```python
from build123d import *
from build123d.topology import SkipClean

# Parameters (mm, degrees)
EXTRUDE1_DEPTH = 4
EXTRUDE2_DEPTH = 3
SKETCH4_R      = 1.5
EXTRUDE3_DEPTH = 4
FILLET3_R      = 3
EXTRUDE4_DEPTH = 4
EXTRUDE6_DEPTH = 3


with BuildPart() as part:
    # Sketch1 → Extrude1 (new body)
    with BuildSketch(Plane.XY):
        Polygon((0, 20.5), (0, 0), (-15, 0), (-15, 10.675), (-1.9, 20.5), align=None)
    extrude(amount=EXTRUDE1_DEPTH)

    # Sketch2 → Extrude2 (cut)
    with BuildSketch(Plane(origin=(0, 0, 0), x_dir=(-1, 0, 0), z_dir=(0, 0, -1))):
        with BuildLine():
            Line((0.4, 14), (0.4, 21.525360588))
            Line((0.4, 21.525360588), (4.6, 21.525360588))
            Line((4.6, 21.525360588), (4.6, 14))
            ThreePointArc((4.6, 14), (2.5, 11.9), (0.4, 14))
        make_face()
    extrude(amount=-EXTRUDE2_DEPTH, mode=Mode.SUBTRACT)

    # Sketch4 → Extrude3 (cut)
    with BuildSketch(Plane.XY.offset(4)):
        with Locations((-3, 8.5)):
            Circle(SKETCH4_R)
        with Locations((-12, 8.5)):
            Circle(SKETCH4_R)
    extrude(amount=-EXTRUDE3_DEPTH, mode=Mode.SUBTRACT)

    # Fillet3
    fillet3_edges = [part.edges().sort_by_distance(p)[0] for p in [
        (0, 0, 2),
    ]]
    fillet(fillet3_edges, radius=FILLET3_R)

    # Sketch5 → Extrude4 (cut)
    with BuildSketch(Plane.XY.offset(4)):
        with BuildLine():
            Line((-1.25, 23.386660478), (-1.25, 17.5))
            ThreePointArc((-1.25, 17.5), (-2.925, 15.825), (-4.6, 17.5))
            Line((-4.6, 17.5), (-4.6, 23.386660478))
            Line((-4.6, 23.386660478), (-1.25, 23.386660478))
        make_face()
    extrude(amount=-EXTRUDE4_DEPTH, mode=Mode.SUBTRACT)

    # Sketch8 → Extrude6 (add)
    with SkipClean():  # the faces are left unmerged after this step: merging them gives an invalid solid
        with BuildSketch(Plane(origin=(0, 0, 0), x_dir=(-1, 0, 0), z_dir=(0, 0, -1))):
            with BuildLine():
                Line((0.4, 20.5), (1.25, 20.5))
                Line((1.25, 20.5), (1.25, 15.687453703))
                ThreePointArc((1.25, 15.687453703), (0.624500067, 14.944722181), (0.4, 14))
                Line((0.4, 14), (0.4, 20.5))
            make_face()
        extrude(amount=-EXTRUDE6_DEPTH)


solid = part.part
```
Here's how the part is built. I have some questions about the finished solid (model axes, mm). A direction names the side the tool comes from. Round coordinates to 2 decimals unless told otherwise and drop trailing zeros. Loops run counter-clockwise (first coordinate to the right, second up) from the corner with the lowest first, then second, coordinate; pieces in that order, holes last. Notation, with made-up numbers: (-11, -22) -> (18, -22) arc R14 ccw to (18, -1) -> close; hole circle Ø1 at (21, 22.5). An arc over 180 degrees is marked (long way). Answer as CSV lines item,"result".
1. If we section it at C-C on y = 18.25: Please give me the cut outline in (x, z), plus the area to 3 significant figures.
Final values:
outline,"(-4.9, 0) -> (-4.6, 0) -> (-4.6, 4) -> (-4.9, 4) -> close; (-1.25, 0) -> (0, 0) -> (0, 4) -> (-1.25, 4) -> close"
area,"6.20 mm^2"
2. Which directions (+Z, -Z, +X, -X, +Y, -Y) give clear straight access to the entire face, cutting with the end or side of a thin tool? Please do faces 4 (the face through (-1.25, 18, 2)), 5 (the face through (0, 12, 2)), 6 (the face through (-3, 14, 3)).
Final values:
face 4,"-Z, +Y"
face 5,"+Z, -Z, +X, +Y, -Y"
face 6,"-Z"
3. Thinking about a two-plate mould opening in X: for faces 1 (the face through (-1, 20.5, 2)), 2 (the face through (-2.31, 7.17, 2.03)), 3 (the face through (-15, 5, 2)), which applies, released by +X, released by -X, zero draft, split by the parting line, or undercut?
Final values:
face 1,"zero draft"
face 2,"undercut"
face 3,"released by -X"
4. If I drill on L1, parallel to X at y = 19.75, z = 2.8; L2, parallel to X at y = 15.75, z = 2.2; L3, parallel to Y at x = -12, z = 1.5 (3 decimals), over which ranges is the centre line in solid material (lowest first)?
Final values:
L1,"x = -1.25 to 0"
L2,"x = -8.23 to -4.6, -1.25 to 0"
L3,"y = 0 to 7, 10 to 12.925"
5. If we section it at B-B on z = 3.7: Please give me the cut outline in (x, y) (3 decimals), plus the area to 3 significant figures.
Final values:
outline,"(-15, 0) -> (-3, 0) arc R3 ccw to (0, 3) -> (0, 20.5) -> (-1.25, 20.5) -> (-1.25, 17.5) arc R1.675 cw to (-4.6, 17.5) -> (-4.6, 18.475) -> (-15, 10.675) -> close; hole circle Ø3 at (-12, 8.5); hole circle Ø3 at (-3, 8.5)"
area,"215 mm^2"
6. For pin 1 (1.3 mm diameter, centred on x = -3.5, y = 13.5, fed in from -Z); pin 2 (1.2 mm diameter, centred on y = 18, z = 2, fed in from -X); pin 3 (2 mm diameter, centred on x = -11.5, z = 2.5, fed in from +Y), each with a flat end and sliding along its axis, tell me the tip position at first contact or that it passes through.
Final values:
pin 1,"stops at z = 3"
pin 2,"stops at x = -6.03"
pin 3,"stops at y = 14.05"
7. If we section it at A-A on y = 8.5: Please give me the cut outline in (x, z).
Final values:
outline,"(-15, 0) -> (-13.5, 0) -> (-13.5, 4) -> (-15, 4) -> close; (-10.5, 0) -> (-4.5, 0) -> (-4.5, 4) -> (-10.5, 4) -> close; (-1.5, 0) -> (0, 0) -> (0, 4) -> (-1.5, 4) -> close"
8. If we section it at D-D on x = -12: Please give me the cut outline in (y, z) (3 decimals), plus the area to 3 significant figures.
Final values:
outline,"(0, 0) -> (7, 0) -> (7, 4) -> (0, 4) -> close; (10, 0) -> (12.925, 0) -> (12.925, 4) -> (10, 4) -> close"
area,"39.7 mm^2"
